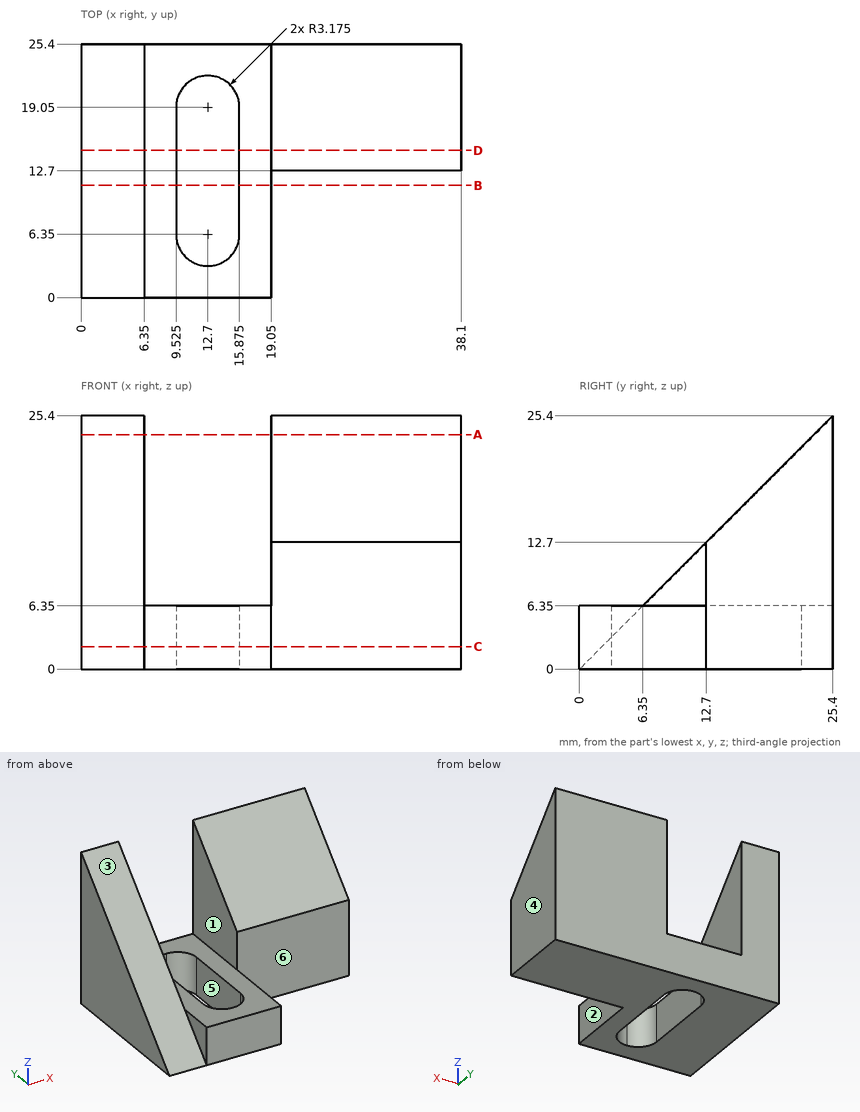
Part print with two shaded views. Sizes in mm from the minimum x, y, z corner. A direction names the side the tool comes from. Round coordinates to 2 decimals unless told otherwise and drop trailing zeros. Loops run counter-clockwise (first coordinate to the right, second up) from the corner with the lowest first, then second, coordinate; pieces in that order, holes last. Notation, with made-up numbers: M 27,49 L 78,49 A21 cw 78,68 Z; hole C 62.5,86.25 d3. An arc over 180 degrees is marked long. Return JSON: item names as keys, results as strings. Group by question number.
(1) Drop flat-ended pins along their axis: P1, Ø4, axis at y = 3, z = 7.5, coming from the -X side; P2, Ø6, axis at x = 21, z = 12.5, coming from the -Y side; P3, Ø1, axis at x = 32.5, y = 12, coming from the -Z side; P4, Ø4, axis at x = 14.5, y = 7, coming from the +Z side. Give the stop position or say it passes through.
(2) Saw through at B-B, the plane y = 11.25. List the corners of the cut face in (x, z) (3 decimals), and give its area (3 significant figures).
(3) Saw through at A-A, the plane z = 23.5. List the corners of the cut face in (x, y), and give its area (3 significant figures).
(4) Mould opens along X. For the marked faces 4, 5 and 6 say: +X half, -X half, draft (parallel to the pull), parting line (faces both ways), or undercut.
(5) Saw through at D-D, the plane y = 14.75. List the corners of the cut face in (x, z) (3 decimals), and give its area (3 significant figures).
(6) Wall check: probe 1 along Z at (x, y) = (8, 6.25); probe 2 along X at (y, z) = (13.5, 5.75) (3 decimals); probe 3 along Y at (x, z) = (30.5, 4). Give the ranges that are in metal, low to high. Write a range as [from, to].
(7) Tool access for the marked faces 1, 2 and 3: list every direction of +Z, -Z, +X, -X, +Y, -Y with a clear straight run to the whole face (end or side of a thin tool).
(8) Saw through at C-C, the plane z = 2.25. List the corners of the cut face in (x, y) (3 decimals).
Answer list:
{
 "1": {"P1": "x = 6.35", "P2": "y = 12.7", "P3": "through", "P4": "z = 6.35"},
 "2": {"outline": "M 0,0 L 9.525,0 L 9.525,6.35 L 6.35,6.35 L 6.35,11.25 L 0,11.25 Z; M 15.875,0 L 19.05,0 L 19.05,6.35 L 15.875,6.35 Z", "area": "112 mm2"},
 "3": {"outline": "M 0,23.5 L 6.35,23.5 L 6.35,25.4 L 0,25.4 Z; M 19.05,23.5 L 38.1,23.5 L 38.1,25.4 L 19.05,25.4 Z", "area": "48.3 mm2"},
 "4": {"face 4": "+X half", "face 5": "undercut", "face 6": "draft"},
 "5": {"outline": "M 0,0 L 9.525,0 L 9.525,6.35 L 6.35,6.35 L 6.35,14.75 L 0,14.75 Z; M 15.875,0 L 38.1,0 L 38.1,14.75 L 19.05,14.75 L 19.05,6.35 L 15.875,6.35 Z", "area": "415 mm2"},
 "6": {"probe 1": "[0, 6.35]", "probe 2": "[0, 9.525], [15.875, 38.1]", "probe 3": "[12.7, 25.4]"},
 "7": {"face 1": "+Z, +Y, -Y", "face 2": "+Z, -Z, +X, -Y", "face 3": "+Z, -X, -Y"},
 "8": {"outline": "M 0,2.25 L 6.35,2.25 L 6.35,0 L 19.05,0 L 19.05,12.7 L 38.1,12.7 L 38.1,25.4 L 0,25.4 Z; hole M 9.525,6.35 A3.175 ccw 15.875,6.35 L 15.875,19.05 A3.175 ccw 9.525,19.05 Z"}
}
